Check sheet for the drawn part. Datum: minimum x, y, z corner. Units: mm. A direction names the side the tool comes from. Give positions to 0.01 mm unless a question says otherwise; leave off trailing zeros. Write each loop counter-clockwise with the first axis right and the second up, starting at its lowest first coordinate (ties: lowest second). Pieces come first, ordered by that corner, then holes. Notation, with made-up numbers: (50.5, 2.25) - (105.5, 2.25) arc R25 ccw to (105.5, 24.25) - close; hole circle Ø5 at (19, 8). An arc over 180 degrees is marked (long way). Use a Markdown table: item, result.
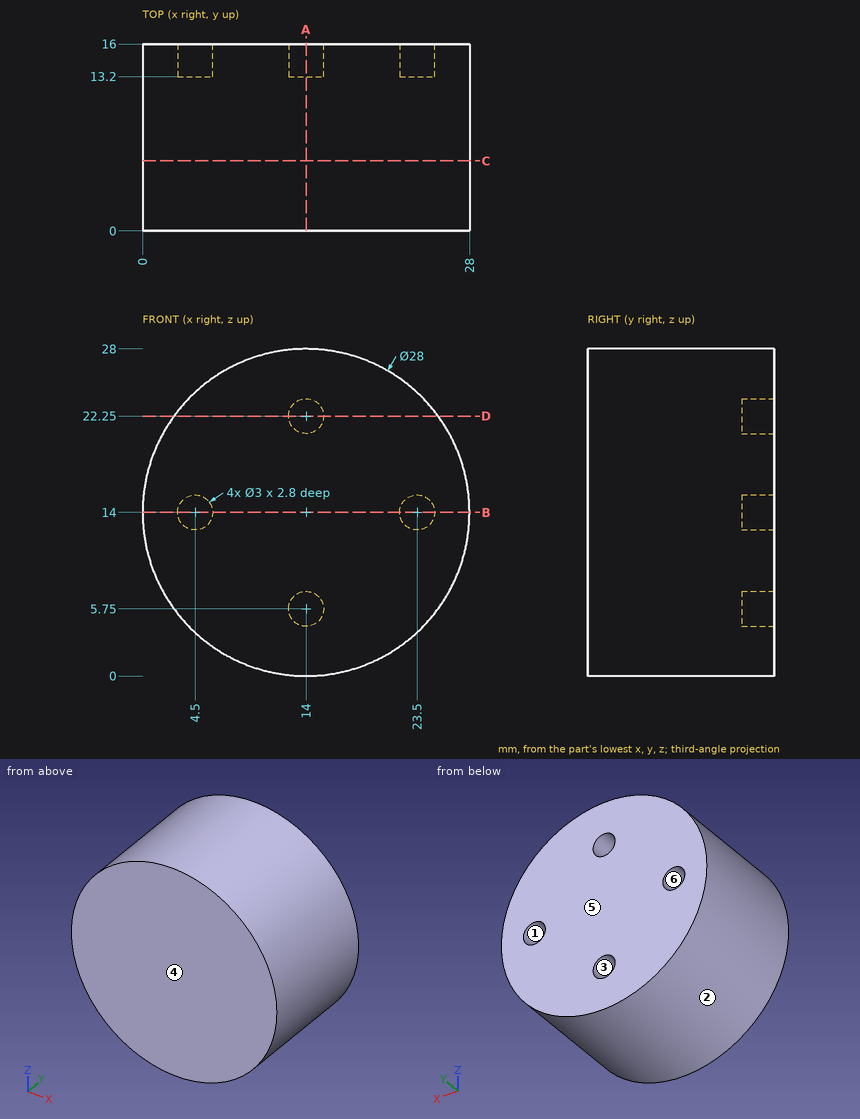
1) Section check C-C on y = 6. Record the boundary of the cut face in (x, z).
Working result:
| item | result |
|---|---|
| outline | circle Ø28 at (14, 14) |
2) Section check D-D on z = 22.25. Record the boundary of the cut face in (x, y).
Working result:
| item | result |
|---|---|
| outline | (2.69, 0) - (25.31, 0) - (25.31, 16) - (15.5, 16) - (15.5, 13.2) - (12.5, 13.2) - (12.5, 16) - (2.69, 16) - close |
3) Section check A-A on x = 14. Record the boundary of the cut face in (y, z).
Working result:
| item | result |
|---|---|
| outline | (0, 0) - (16, 0) - (16, 4.25) - (13.2, 4.25) - (13.2, 7.25) - (16, 7.25) - (16, 20.75) - (13.2, 20.75) - (13.2, 23.75) - (16, 23.75) - (16, 28) - (0, 28) - close |
4) Section check B-B on z = 14. Record the boundary of the cut face in (x, y).
Working result:
| item | result |
|---|---|
| outline | (0, 0) - (28, 0) - (28, 16) - (25, 16) - (25, 13.2) - (22, 13.2) - (22, 16) - (6, 16) - (6, 13.2) - (3, 13.2) - (3, 16) - (0, 16) - close |
5) Depth check by flat-ended pin: P1, Ø6, axis at y = 5, z = 17.5, coming from the -X side; P2, Ø6, axis at x = 24.5, y = 6, coming from the -Z side; P3, Ø0.9, axis at x = 14.5, z = 5, coming from the +Y side. Enter the tip coordinate at first touch or a pass-through.
Working result:
| item | result |
|---|---|
| P1 | stops at x = 0.01 |
| P2 | stops at z = 2.18 |
| P3 | stops at y = 13.2 |
6) Mould release check, pull along Z, two halves, no side actions. Record for the marked faces 1, 2, 3 and 4: pulls with the +Z half, pulls with the -Z half, needs draft (parallel to the pull), parting line crosses it, or undercut.
Working result:
| item | result |
|---|---|
| face 1 | undercut |
| face 2 | parting line crosses it |
| face 3 | undercut |
| face 4 | needs draft |
7) Set-up check for the marked faces 5 and 6: record each of +Z, -Z, +X, -X, +Y, -Y from which the full face is reachable in a straight line by a thin tool's end or side.
Working result:
| item | result |
|---|---|
| face 5 | +Z, -Z, +X, -X, +Y |
| face 6 | +Y |
8) Material ranges on L1, parallel to Z at x = 14, y = 13.8; L2, parallel to Z at x = 4.5, y = 14.7; L3, parallel to Z at x = 14, y = 6.5, recorded low to high. Write a range as from..to.
Working result:
| item | result |
|---|---|
| L1 | z = 0..4.25, 7.25..20.75, 23.75..28 |
| L2 | z = 3.72..12.5, 15.5..24.28 |
| L3 | z = 0..28 |
